```python
from build123d import *

# Parameters (mm, degrees)
SKETCH2_W           = 110
SKETCH2_H           = 110
SKETCH2_R           = 1.6
SKETCH2_R_2         = 10
BOSS_EXTRUDE1_DEPTH = 3
FILLET1_R           = 10


with BuildPart() as part:
    # Sketch2 → Boss-Extrude1 (new body)
    with BuildSketch(Plane(origin=(0, 0, 0), x_dir=(1, 0, 0), z_dir=(0, 1, 0))):
        Rectangle(SKETCH2_W, SKETCH2_H)
        with Locations(Location((15.25, 15.25, 0), (0, 0, 270))):
            Circle(SKETCH2_R, mode=Mode.SUBTRACT)
        with Locations(Location((-15.25, 15.25, 0), (0, 0, 90))):
            Circle(SKETCH2_R, mode=Mode.SUBTRACT)
        with Locations(Location((-15.25, -15.25, 0), (0, 0, 270))):
            Circle(SKETCH2_R, mode=Mode.SUBTRACT)
        with Locations(Location((15.25, -15.25, 0), (0, 0, 90))):
            Circle(SKETCH2_R, mode=Mode.SUBTRACT)
        with Locations(Location((35.3553, 35.3553, 0), (0, 0, 270))):
            Circle(SKETCH2_R, mode=Mode.SUBTRACT)
        with Locations(Location((45.9619, 45.9619, 0), (0, 0, 270))):
            Circle(SKETCH2_R, mode=Mode.SUBTRACT)
        with Locations(Location((-35.3553, 35.3553, 0), (0, 0, 90))):
            Circle(SKETCH2_R, mode=Mode.SUBTRACT)
        with Locations(Location((-45.9619, 45.9619, 0), (0, 0, 90))):
            Circle(SKETCH2_R, mode=Mode.SUBTRACT)
        with Locations(Location((45.9619, -45.9619, 0), (0, 0, 90))):
            Circle(SKETCH2_R, mode=Mode.SUBTRACT)
        with Locations(Location((35.3553, -35.3553, 0), (0, 0, 90))):
            Circle(SKETCH2_R, mode=Mode.SUBTRACT)
        with Locations(Location((-45.9619, -45.9619, 0), (0, 0, 270))):
            Circle(SKETCH2_R, mode=Mode.SUBTRACT)
        with Locations(Location((-35.3553, -35.3553, 0), (0, 0, 270))):
            Circle(SKETCH2_R, mode=Mode.SUBTRACT)
        with Locations(Location((0, 45, 0), (0, 0, 270))):
            Circle(SKETCH2_R, mode=Mode.SUBTRACT)
        with Locations(Location((0, -45, 0), (0, 0, 270))):
            Circle(SKETCH2_R, mode=Mode.SUBTRACT)
        with Locations(Location((45, 0, 0), (0, 0, 270))):
            Circle(SKETCH2_R, mode=Mode.SUBTRACT)
        with Locations(Location((-45, 0, 0), (0, 0, 270))):
            Circle(SKETCH2_R, mode=Mode.SUBTRACT)
        with Locations(Location((0, 0, 0), (0, 0, 270))):
            Circle(SKETCH2_R_2, mode=Mode.SUBTRACT)
    extrude(amount=BOSS_EXTRUDE1_DEPTH)

    # Fillet1
    fillet1_edges = [part.edges().sort_by_distance(p)[0] for p in [
        (55, 1.5, 55),
        (-55, 1.5, 55),
        (-55, 1.5, -55),
        (55, 1.5, -55),
    ]]
    fillet(fillet1_edges, radius=FILLET1_R)


solid = part.part
```
Verification items for the finished model (mm, model axes). Round coordinates to 2 decimals unless told otherwise and drop trailing zeros. Write each loop counter-clockwise with the first axis right and the second up, starting at its lowest first coordinate (ties: lowest second). Pieces come first, ordered by that corner, then holes. Notation, with made-up numbers: (74, 12) - (90, 12) arc R16 ccw to (90, 41) - close; hole circle Ø8 at (32.5, 72.25). An arc over 180 degrees is marked (long way). Answer as a JSON object with one key per item and string values. Group by question number.
Q1. Section check A-A, the plane x = 0. Enter the section's corners in (y, z).
Q2. Mould release check, pull along Z, two halves, no side actions. Record for faces 1 (the flat face through (-1, 1, 55)), 2 (the cylindrical face through (-52.15, 1.52, -51.99)), 3 (the cylindrical face through (-47.38, 1.48, 46.7)): released by +Z, released by -Z, zero draft, split by the parting line, or undercut.
Q3. Section check B-B, the plane z = 15.25. Enter the section's corners in (x, y).
Q4. Section check D-D, the plane z = 0. Enter the section's corners in (x, y).
Q5. Thickness scan on line 1 (X direction, y = 1.8, z = 0); line 2 (X direction, y = 1.7, z = 15.25); line 3 (Z direction, x = -14, y = 2.35). Record the ranges inside material, lowest first.
Q6. Section check C-C, the plane x = -15.25. Enter the section's corners in (y, z), plus the area to 3 significant figures.
Found:
{
 "1": {"outline": "(0, -55) - (3, -55) - (3, -46.6) - (0, -46.6) - close; (0, -43.4) - (3, -43.4) - (3, -10) - (0, -10) - close; (0, 10) - (3, 10) - (3, 43.4) - (0, 43.4) - close; (0, 46.6) - (3, 46.6) - (3, 55) - (0, 55) - close"},
 "2": {"face 1": "released by +Z", "face 2": "released by -Z", "face 3": "undercut"},
 "3": {"outline": "(-55, 0) - (-16.85, 0) - (-16.85, 3) - (-55, 3) - close; (-13.65, 0) - (13.65, 0) - (13.65, 3) - (-13.65, 3) - close; (16.85, 0) - (55, 0) - (55, 3) - (16.85, 3) - close"},
 "4": {"outline": "(-55, 0) - (-46.6, 0) - (-46.6, 3) - (-55, 3) - close; (-43.4, 0) - (-10, 0) - (-10, 3) - (-43.4, 3) - close; (10, 0) - (43.4, 0) - (43.4, 3) - (10, 3) - close; (46.6, 0) - (55, 0) - (55, 3) - (46.6, 3) - close"},
 "5": {"line 1": "x = -55 to -46.6, -43.4 to -10, 10 to 43.4, 46.6 to 55", "line 2": "x = -55 to -16.85, -13.65 to 13.65, 16.85 to 55", "line 3": "z = -55 to -16.25, -14.25 to 14.25, 16.25 to 55"},
 "6": {"outline": "(0, -55) - (3, -55) - (3, -16.85) - (0, -16.85) - close; (0, -13.65) - (3, -13.65) - (3, 13.65) - (0, 13.65) - close; (0, 16.85) - (3, 16.85) - (3, 55) - (0, 55) - close", "area": "311 mm^2"}
}
